Build history of the part. All positions in model axes, mm. Face numbers are marked on the shaded views. Give positions to 0.01 mm unless a question says otherwise; leave off trailing zeros. Write each loop counter-clockwise with the first axis right and the second up, starting at its lowest first coordinate (ties: lowest second). Pieces come first, ordered by that corner, then holes. Notation, with made-up numbers: M -34.5,76.25 L -2.5,76.25 A15 cw -2.5,83.25 Z; hole C 62.5,-22 d4. An arc over 180 degrees is marked long. One line per item, written item: value. Start each with the question number.
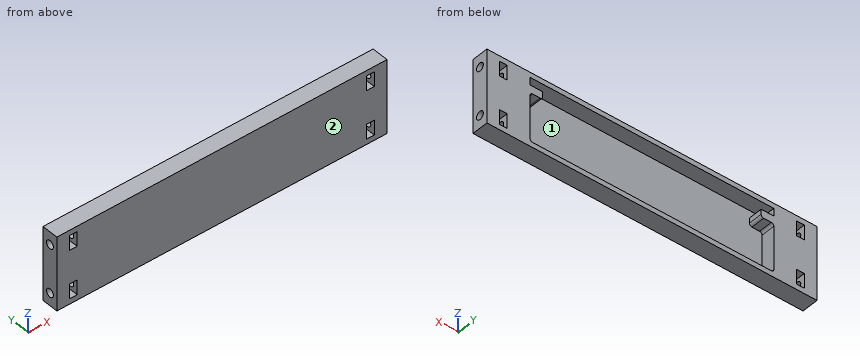
from build123d import *

# Parameters (mm, degrees)
CROQUIS1_W              = 130
CROQUIS1_H              = 29
SALIENTE_EXTRUIR1_DEPTH = 6.5
CORTAR_EXTRUIR1_DEPTH   = 5.5
CROQUIS3_W              = 3
CROQUIS3_H              = 5.8
CORTAR_EXTRUIR2_DEPTH   = 67.91412407
CROQUIS4_R              = 1.6
CORTAR_EXTRUIR3_DEPTH   = 15
CORTAR_EXTRUIR4_START   = -15
CROQUIS5_R              = 1.6
CORTAR_EXTRUIR4_DEPTH   = 15
REDONDEO1_R             = 1


with BuildPart() as part:
    # Croquis1 → Saliente-Extruir1 (new body)
    with BuildSketch(Plane(origin=(0, 0, 0), x_dir=(1, 0, 0), z_dir=(0, 1, 0))):
        Rectangle(CROQUIS1_W, CROQUIS1_H)
    extrude(amount=SALIENTE_EXTRUIR1_DEPTH)

    # Croquis2 → Cortar-Extruir1 (cut)
    with BuildSketch(Plane(origin=(0, 6.5, 0), x_dir=(1, 0, 0), z_dir=(0, 1, 0))):
        Polygon((48, 12.5), (-48, 12.5), (-48, -6.5), (-43, -6.5), (-43, -9.5), (-48, -9.5), (-48, -12.5), (48, -12.5), (48, -9.5), (43, -9.5), (43, -6.5), (48, -6.5), align=None)
    extrude(amount=-CORTAR_EXTRUIR1_DEPTH, mode=Mode.SUBTRACT)

    # Croquis3 → Cortar-Extruir2 (cut, through all)
    with BuildSketch(Plane(origin=(0, 6.5, 0), x_dir=(1, 0, 0), z_dir=(0, 1, 0))):
        with Locations((-58.5, -9.5)):
            Rectangle(CROQUIS3_W, CROQUIS3_H)
        with Locations((-58.5, 9.5)):
            Rectangle(CROQUIS3_W, CROQUIS3_H)
        with Locations((58.5, -9.5)):
            Rectangle(CROQUIS3_W, CROQUIS3_H)
        with Locations((58.5, 9.5)):
            Rectangle(CROQUIS3_W, CROQUIS3_H)
    extrude(amount=-CORTAR_EXTRUIR2_DEPTH, mode=Mode.SUBTRACT)

    # Croquis4 → Cortar-Extruir3 (cut)
    with BuildSketch(Plane.ZY.offset(65)):
        with Locations((-9.5, 3.25)):
            Circle(CROQUIS4_R)
        with Locations(Location((9.5, 3.25, 0), (0, 0, 180))):
            Circle(CROQUIS4_R)
    extrude(amount=-CORTAR_EXTRUIR3_DEPTH, mode=Mode.SUBTRACT)

    # Croquis5 → Cortar-Extruir4 (cut)
    with BuildSketch(Plane(origin=(65, 0, 0), x_dir=(0, 0, -1), z_dir=(1, 0, 0)).offset(CORTAR_EXTRUIR4_START)):
        with Locations((-9.5, 3.25)):
            Circle(CROQUIS5_R)
        with Locations(Location((9.5, 3.25, 0), (0, 0, 180))):
            Circle(CROQUIS5_R)
    extrude(amount=CORTAR_EXTRUIR4_DEPTH, mode=Mode.SUBTRACT)

    # Redondeo1
    redondeo1_edges = [part.edges().sort_by_distance(p)[0] for p in [
        (-48, 3.75, 6.5),
        (-48, 3.75, -12.5),
        (48, 3.75, -12.5),
        (48, 3.75, 6.5),
        (43, 3.75, 6.5),
        (-43, 3.75, 6.5),
    ]]
    fillet(redondeo1_edges, radius=REDONDEO1_R)


solid = part.part
1) Probe line 1 along Z through (x, y) = (47, 1.75); line 2 along X through (y, z) = (4.75, 8.25); line 3 along Z through (x, y) = (53.5, 3.25). List the from-to ranges inside material, lowest first. Write a range as from..to.
2) Mould opens along Z. For the marked faces 1 and 2 say: released by +Z, released by -Z, zero draft, split by the parting line, or undercut.
3) Band-saw the part on A-A (z = -9.5). Count the separate pieces of the cut face and the enclosed holes in it, then the cut area to 3 significant figures.
4) Band-saw the part on B-B (z = 0.75). List the corners of the cut face in (x, y).
5) Drop flat-ended pins along their axis: P1, Ø8, axis at x = -8, z = -7, coming from the +Y side; P2, Ø1.9, axis at y = 3.25, z = 9.5, coming from the +X side. Give the stop position or say it passes through.
6) Band-saw the part on C-C (x = 23). List the corners of the cut face in (y, z).
Model answer:
1. line 1: z = -14.5..-12.5, 6.5..9.5, 12.5..14.5
1. line 2: x = -65..-60, -57..-43, 43..57, 60..65
1. line 3: z = -14.5..-11.1, -7.9..7.9, 11.1..14.5
2. face 1: undercut
2. face 2: zero draft
3. separate pieces: 5
3. enclosed holes: 0
3. area: 201 mm²
4. outline: M -65,0 L 65,0 L 65,6.5 L 48,6.5 L 48,1 L -48,1 L -48,6.5 L -65,6.5 Z
5. P1: stops at y = 1
5. P2: stops at x = 50
6. outline: M 0,-14.5 L 6.5,-14.5 L 6.5,-12.5 L 1,-12.5 L 1,12.5 L 6.5,12.5 L 6.5,14.5 L 0,14.5 Z
